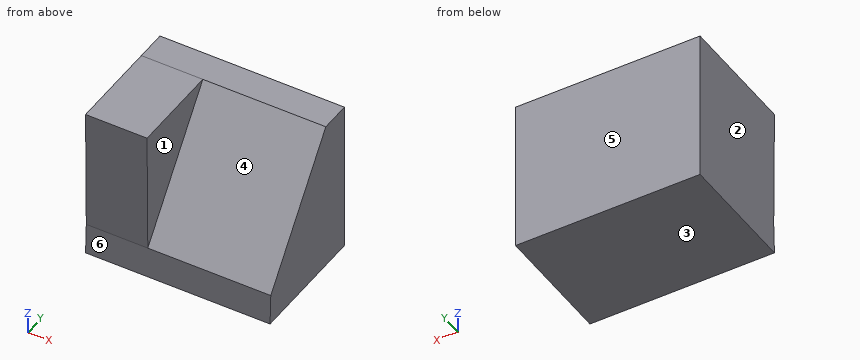
```python
from build123d import *

# Parameters (mm, degrees)
F1_DEPTH = 38.1
F3_DEPTH = 12.7


with BuildPart() as f1:
    # F0 (on Right) → F1 (new body)
    with BuildSketch(Plane.YZ):
        Polygon((-54.048603, -35.997721), (-54.302403, -42.342647), (-28.902403, -42.342647), (-28.902403, -10.592647), (-35.252403, -10.592647), align=None)
    extrude(amount=F1_DEPTH)

    # F2 (on face) → F3 (join)
    with BuildSketch(Plane(origin=(0, 0, 0), x_dir=(0, -1, 0), z_dir=(-1, 0, 0))):
        Polygon((54.302402, -10.598989), (35.252403, -10.592647), (54.048603, -35.997721), align=None)
    extrude(amount=-F3_DEPTH)


solid = f1.part
```
Check sheet for the modelled part. Datum: model origin and axes. Units: mm. Face numbers are marked on the shaded views. A direction names the side the tool comes from. Round coordinates to 2 decimals unless told otherwise and drop trailing zeros. Order: outer loops, then holes, each group sorted by start corner. A loop starts at its lowest first (then second) coordinate and runs counter-clockwise, first axis right, second up. Notation, with made-up numbers: (-3.75, 71.5) - (18.25, 71.5) arc R13 ccw to (18.25, 75.5) - close; hole circle Ø4 at (-39.75, 51). An arc over 180 degrees is marked (long way). Answer as CSV lines item,"result". Start each with the question number.
1) Draft check along Z on the marked faces 3, 4, 5 and 6. Enter one of: +Z half, -Z half, draft (parallel to the pull), parting line (faces both ways), or undercut.
2) Tool access check on the marked faces 1 and 2. Record the directions out of +Z, -Z, +X, -X, +Y, -Y that give a thin tool (end or side, any length) a straight path to the whole face; none if there is none.
3) Section check C-C (z = -14.5). Record the cut outline in (x, y).
4) Depth check by flat-ended pin: pin 1 (4 mm diameter, centred on x = 19, z = -36.5, fed in from -Y); pin 2 (5 mm diameter, centred on x = 13, z = -20, fed in from -Y); pin 3 (8 mm diameter, centred on x = 24.5, z = -17, fed in from -Y). Enter the tip coordinate at first touch or a pass-through.
5) Scan lines: probe 1 along X at (y, z) = (-43, -16); probe 2 along Z at (x, y) = (13.5, -37.5); probe 3 along Y at (x, z) = (20, -26). Record each from-to range of solid material in increasing order.
6) Section check A-A (x = 33.5). Record the cut outline in (y, z).
7) Section check B-B (y = -43.5). Record the cut outline in (x, z).
Determined:
1,face 3,"-Z half"
1,face 4,"+Z half"
1,face 5,"draft"
1,face 6,"undercut"
2,face 1,"+Z, +X, -Y"
2,face 2,"+Z, -Z, -X, +Y, -Y"
3,outline,"(0, -54.26) - (12.7, -54.26) - (12.7, -38.14) - (38.1, -38.14) - (38.1, -28.9) - (0, -28.9) - close"
4,pin 1,"y = -54.15"
4,pin 2,"y = -54.23"
4,pin 3,"y = -42.95"
5,probe 1,"0 to 12.7"
5,probe 2,"-42.34 to -13.63"
5,probe 3,"-46.65 to -28.9"
6,outline,"(-54.3, -42.34) - (-28.9, -42.34) - (-28.9, -10.59) - (-35.25, -10.59) - (-54.05, -36) - close"
7,outline,"(0, -42.34) - (38.1, -42.34) - (38.1, -21.74) - (12.7, -21.74) - (12.7, -10.6) - (0, -10.6) - close"
